Autodesk Inventor part; units mm, degrees
ref_plane "fix_end_l_XY" through (0, 17, 0) normal (0, 0, 1) x (1, 0, 0)
ref_plane "fix_end_l_YZ" through (0, 17, 0) normal (1, 0, 0) x (0, 1, 0)
ref_plane "fix_end_l_ZX" through (0, 17, 0) normal (0, 1, 0) x (0, 0, 1)
sketch "Sketch_1" plane through (0, 0, 0) normal (0, 0, 1) x (1, 0, 0)
  arc A0 (-16.7417, 19.952) -> (-16.7417, 14.048) centre (0, 17) ccw
  line L0 (-16.7417, 14.048) -> (-7.3861, 15.6976)
  arc A1 (-7.3861, 15.6976) -> (-5.3033, 11.6967) centre (0, 17) ccw
  line L1 (-5.3033, 11.6967) -> (-12.0208, 4.9792)
  arc A2 (-12.0208, 4.9792) -> (0, 0) centre (0, 17) ccw
  line L2 (0, 0) -> (60, 0)
  line L3 (60, 0) -> (60, 4.67)
  arc A3 (60, 4.67) -> (58.0834, 7.7293) centre (56.6, 4.67) ccw
  line L4 (58.0834, 7.7293) -> (7.4171, 32.2966)
  arc A4 (7.4171, 32.2966) -> (-12.0208, 29.0208) centre (0, 17) ccw
  line L5 (-12.0208, 29.0208) -> (-5.3033, 22.3033)
  arc A5 (-5.3033, 22.3033) -> (-7.3861, 18.3024) centre (0, 17) ccw
  line L6 (-7.3861, 18.3024) -> (-16.7417, 19.952)
  circle A6 centre (0, 17) radius 4.25
extrude "Extrusion1" add sketch "Sketch_1" against normal blind 20
sketch "Sketch_2" plane through (0, 0, 0) normal (1, 0, 0) x (0, 1, 0)
  line L0 (39, 5) -> (-5, 5)
  line L1 (-5, 5) -> (-5, -25)
  line L2 (-5, -25) -> (39, -25)
  line L3 (39, -25) -> (39, 5)
  arc A0 (2, 0) -> (0, -2) centre (2, -2) ccw
  line L4 (0, -2) -> (0, -20)
  line L5 (0, -20) -> (2, -20)
  line L6 (2, -20) -> (2, -3)
  arc A1 (3, -2) -> (2, -3) centre (3, -3) ccw
  line L7 (3, -2) -> (34, -2)
  line L8 (34, -2) -> (34, 0)
  line L9 (34, 0) -> (2, 0)
extrude "Extrusion2" cut sketch "Sketch_2" along normal mid plane 120
sketch "Sketch_3" plane through (0, 0, 0) normal (0, 1, 0) x (-1, 0, 0)
  line L0 (22, -25) -> (22, 5)
  line L1 (22, 5) -> (-65, 5)
  line L2 (-65, 5) -> (-65, -25)
  line L3 (-65, -25) -> (22, -25)
  line L4 (17, -2) -> (17, 0)
  line L5 (17, 0) -> (-60, 0)
  line L6 (-60, 0) -> (-60, -15)
  arc A0 (-60, -15) -> (-55, -20) centre (-55, -15) ccw
  line L7 (-55, -20) -> (-25, -20)
  arc A1 (-25, -20) -> (-20, -15) centre (-25, -15) ccw
  line L8 (-20, -15) -> (-20, -2)
  line L9 (-20, -2) -> (17, -2)
extrude "Extrusion3" cut sketch "Sketch_3" along normal blind 34
sketch "Sketch4" plane through (20, 0, -2) normal (0, -1, 0) x (1, 0, 0)
  point P0 (8, -8)
hole "Hole1" at (28, 0, -10) direction (0, 1, 0) diameter 7 depth 2
sketch "Sketch5" plane through (20, 0, -2) normal (0, -1, 0) x (1, 0, 0)
  point P0 (32, -8)
hole "Hole2" at (52, 0, -10) direction (0, 1, 0) diameter 7 depth 2
sketch "Sketch_7" plane through (0, 0, 0) normal (0, 0, 1) x (1, 0, 0)
  circle A0 centre (15, 0) radius 2.5
extrude "Extrusion4" cut sketch "Sketch_7" against normal blind 20
ref_plane "fix_end_l_XY" through (0, 17, 0) normal (0, 0, 1) x (1, 0, 0)
ref_plane "fix_end_l_YZ" through (0, 17, 0) normal (1, 0, 0) x (0, 1, 0)
ref_plane "fix_end_l_ZX" through (0, 17, 0) normal (0, 1, 0) x (0, 0, 1)
ref_plane "free_end_l_XY" through (0, 17, -2) normal (0, 0, 1) x (1, 0, 0)
ref_plane "free_end_l_YZ" through (0, 17, -2) normal (1, 0, 0) x (0, 1, 0)
ref_plane "free_end_l_ZX" through (0, 17, -2) normal (0, 1, 0) x (0, 0, 1)
ref_plane "l_to_r_XY" through (0, 17, -26) normal (0, 0, 1) x (1, 0, 0)
ref_plane "l_to_r_YZ" through (0, 17, -26) normal (1, 0, 0) x (0, 1, 0)
ref_plane "l_to_r_ZX" through (0, 17, -26) normal (0, 1, 0) x (0, 0, 1)
ref_plane "to_clip1_XY" through (0, 17, -10) normal (1, 0, 0) x (0, 0, -1)
ref_plane "to_clip1_YZ" through (0, 17, -10) normal (0, 0, -1) x (0, 1, 0)
ref_plane "to_clip1_ZX" through (0, 17, -10) normal (0, 1, 0) x (1, 0, 0)
properties part number "MHPUS306-Ab_fixed_left"
Model file for the job. Use its own axes, mm. A direction names the side the tool comes from. Give positions to 0.01 mm unless a question says otherwise; leave off trailing zeros. Loops run counter-clockwise (first coordinate to the right, second up) from the corner with the lowest first, then second, coordinate; pieces in that order, holes last. Notation, with made-up numbers: (75.25, 68) - (97.25, 68) arc R6 cw to (97.25, 73) - close; hole circle Ø5 at (-8.5, -16.75). An arc over 180 degrees is marked (long way). One line per item, written item: value. Start each with the question number.
1. Slice it at A-A (z = -10). List the corners of the cut face in (x, y).
2. Slice it at C-C (y = 17). List the corners of the cut face in (x, z), plus the area to 3 significant figures.
3. Which spindle directions (+Z, -Z, +X, -X, +Y, -Y) get a long thin tool onto all of the face, cutting with end or side? Do faces 1 (the cylindrical face through (-2.68, 33.787, -0.986)), 2 (the flat face through (-9, 8, -1)), 3 (the cylindrical face through (-6.67, 13.57, -0.99)). Say none if no direction does.
4. Pin check, flat tips, straight feed: pin 1 (0.9 mm diameter, centred on y = 1, z = -9.5, fed in from -X); pin 2 (8 mm diameter, centred on x = 50, z = -5.5, fed in from +Y); pin 3 (17 mm diameter, centred on x = 16, y = 21, fed in from -Z). Stop position of each tip, or through.
5. Slice it at B-B (x = 28). List the corners of the cut face in (y, z).
6. Pull direction X, two halves, no side cores. Call faces 4 (the flat face through (-11.998, 19.116, -0.986)), 5 (the cylindrical face through (4.99, 0.57, -0.6)), 6 (the flat face through (-9, 26, -1)), 7 (the cylindrical face through (-0.92, 12.85, -0.99)): pulls with the +X half, pulls with the -X half, needs draft (parallel to the pull), parting line crosses it, or undercut.
7. Probe L1, parallel to X at y = 0.75, z = -10; L2, parallel to Z at x = 32.5, y = 5.5; L3, parallel to Y at x = 38, z = -7.5. List the from-to ranges inside material, lowest first. Write a range as from..to.
8. Slice it at D-D (x = -1). List the corners of the cut face in (y, z), plus the area to 3 significant figures.
Solution:
1. outline: (20, 0) - (24.5, 0) - (24.5, 2) - (20, 2) - close; (31.5, 0) - (48.5, 0) - (48.5, 2) - (31.5, 2) - close; (55.5, 0) - (60, 0) - (60, 2) - (55.5, 2) - close
2. outline: (-17, -2) - (-4.25, -2) - (-4.25, 0) - (-17, 0) - close; (4.25, -2) - (38.96, -2) - (38.96, 0) - (4.25, 0) - close
2. area: 94.9 mm^2
3. face 1: +Z, -Z, +Y
3. face 2: +Z, -Z, -X
3. face 3: +Z, -Z
4. pin 1: stops at x = 20
4. pin 2: stops at y = 12.59
4. pin 3: stops at z = -2
5. outline: (0, -20) - (2, -20) - (2, -13.5) - (0, -13.5) - close; (0, -6.5) - (2, -6.5) - (2, -3) arc R1 cw to (3, -2) - (22.32, -2) - (22.32, 0) - (2, 0) arc R2 ccw to (0, -2) - close
6. face 4: undercut
6. face 5: needs draft
6. face 6: pulls with the -X half
6. face 7: undercut
7. L1: x = 20..24.5, 31.5..48.5, 55.5..60
7. L2: z = -2..0
7. L3: y = 0..2
8. outline: (0.03, -2) - (12.87, -2) - (12.87, 0) - (2, 0) arc R2 ccw to (0.03, -1.66) - close; (21.13, -2) - (33.97, -2) - (33.97, 0) - (21.13, 0) - close
8. area: 50.6 mm^2
